from build123d import *

# Parameters (mm, degrees)
F0_R     = 6.35
F1_DEPTH = 6.35


with BuildPart() as f1:
    # F0 (on Front) → F1 (new body)
    with BuildSketch(Plane.XZ):
        with BuildLine():
            ThreePointArc((24.967043, 5.047776), (27.078139, 12.979448), (33.599452, 17.963487))
            ThreePointArc((33.599452, 17.963487), (32.995568, 19.05), (32.356562, 20.116235))
            ThreePointArc((32.356562, 20.116235), (24.779601, 16.960632), (16.855024, 19.098206))
            ThreePointArc((16.855024, 19.098206), (0, 12.7), (-16.855024, 19.098206))
            ThreePointArc((-16.855024, 19.098206), (-24.779601, 16.960632), (-32.356562, 20.116235))
            ThreePointArc((-32.356562, 20.116235), (-32.995568, 19.05), (-33.599452, 17.963487))
            ThreePointArc((-33.599452, 17.963487), (-27.327541, 13.339033), (-24.936894, 5.922346))
            ThreePointArc((-24.936894, 5.922346), (-24.944434, 5.484801), (-24.967043, 5.047776))
            ThreePointArc((-24.967043, 5.047776), (-12.391144, -4.196794), (-7.595568, -19.05))
            ThreePointArc((-7.595568, -19.05), (-7.725011, -21.611042), (-8.11202, -24.145982))
            ThreePointArc((-8.11202, -24.145982), (-2.916324, -28.830524), (-0.989545, -35.55568))
            ThreePointArc((-0.989545, -35.55568), (-1.05304, -36.824042), (-1.24289, -38.079722))
            ThreePointArc((-1.24289, -38.079722), (0, -38.1), (1.24289, -38.079722))
            ThreePointArc((1.24289, -38.079722), (2.298538, -29.94008), (8.11202, -24.145982))
            ThreePointArc((8.11202, -24.145982), (10.998523, -6.35), (24.967043, 5.047776))
        make_face()
        Circle(F0_R, mode=Mode.SUBTRACT)
    extrude(amount=F1_DEPTH)


solid = f1.part
Source: CAD feature listing. Evaluate the final solid. Frame: model axes, mm. A direction names the side the tool comes from. Give positions to 0.01 mm unless a question says otherwise; leave off trailing zeros. Write each loop counter-clockwise with the first axis right and the second up, starting at its lowest first coordinate (ties: lowest second). Pieces come first, ordered by that corner, then holes. Notation, with made-up numbers: M 57,58.25 L 106,58.25 A29 ccw 106,84.25 Z; hole C 21.25,71 d4. An arc over 180 degrees is marked long. Return JSON: item names as keys, results as strings. Group by question number.
1) Ray query, L1, parallel to Z at x = 0, y = -3.75; L2, parallel to Z at x = -3.5, y = -2; L3, parallel to X at y = -0.75, z = -33. Return the intervals inside material, ascending.
2) First-contact query: pin 1 Ø2 at (x, y) = (-6.5, -1.5) entering from +Z; pin 2 Ø1 at (y, z) = (-4.5, -8) entering from -X; pin 3 Ø12 at (x, z) = (10, -30.5) entering from +Y; pin 4 Ø2 at (y, z) = (-5.5, 9.5) entering from -X. Flat tips, straight axial feed; report the tip coordinate or a pass-through.
3) Cut plane B-B, the plane x = 0. Output: boundary loops of the cut face in (y, z).
4) Cut plane C-C, the plane z = 0. Output: boundary loops of the cut face in (x, y), then the cut area to 3 significant figures.
5) Cut plane D-D, the plane z = -10. Output: boundary loops of the cut face in (x, y), then the cut area to 3 significant figures.
6) Cut plane A-A, the plane y = -2. Output: boundary loops of the cut face in (x, z), then the cut area to 3 significant figures.
7) Set-up query: faces 4 (the face through (-5.1, 0, 4.1)), 5 (the face through (-1.05, -3.13, -36.81)). Return all of +Z, -Z, +X, -X, +Y, -Y with unobstructed straight access to the full face (end or side cutting, diameter ignored); none if empty.
8) Draft query along Z for faces 1 (the face through (-3, -3.1, -28.7)), 2 (the face through (0, -3.1, -38.1)), 3 (the face through (-24.663, -3.131, 16.954)). Return one class per face: released by +Z, released by -Z, zero draft, split by the parting line, or undercut.
Data:
{
 "1": {"L1": "z = -38.1 to -6.35, 6.35 to 12.7", "L2": "z = -27.98 to -5.3, 5.3 to 12.94", "L3": "x = -1.25 to 1.25"},
 "2": {"pin 1": "stops at z = 13.83", "pin 2": "stops at x = -10.37", "pin 3": "passes through", "pin 4": "stops at x = -25.79"},
 "3": {"outline": "M -6.35,-38.1 L 0,-38.1 L 0,-6.35 L -6.35,-6.35 Z; M -6.35,6.35 L 0,6.35 L 0,12.7 L -6.35,12.7 Z"},
 "4": {"outline": "M -16.2,-6.35 L -6.35,-6.35 L -6.35,0 L -16.2,0 Z; M 6.35,-6.35 L 16.2,-6.35 L 16.2,0 L 6.35,0 Z", "area": "125 mm²"},
 "5": {"outline": "M -9.26,-6.35 L 9.26,-6.35 L 9.26,0 L -9.26,0 Z", "area": "118 mm²"},
 "6": {"outline": "M -33.6,17.96 A12.7 cw -24.94,5.92 A12.7 cw -24.97,5.05 A25.4 cw -7.6,-19.05 A25.4 cw -8.11,-24.15 A12.7 cw -0.99,-35.56 A12.7 cw -1.24,-38.08 A38.1 ccw 1.24,-38.08 A12.7 cw 8.11,-24.15 A25.4 cw 24.97,5.05 A12.7 cw 33.6,17.96 A38.1 ccw 32.36,20.12 A12.7 cw 16.86,19.1 A25.4 cw -16.86,19.1 A12.7 cw -32.36,20.12 A38.1 ccw Z; hole C 0,0 d12.7", "area": "1,210 mm²"},
 "7": {"face 4": "+Z, -Z, +X, -X, +Y", "face 5": "-X, +Y, -Y"},
 "8": {"face 1": "undercut", "face 2": "released by -Z", "face 3": "released by +Z"}
}
